```python
from build123d import *

# Parameters (mm, degrees)
SKETCH1_R           = 21
SKETCH1_R_2         = 15.5
SKETCH1_R_3         = 1.5
BOSS_EXTRUDE1_DEPTH = 3
SKETCH2_R           = 2.5
BOSS_EXTRUDE2_DEPTH = 29
CUT_EXTRUDE1_START  = -5
SKETCH3_R           = 1.5
CUT_EXTRUDE1_DEPTH  = 5


with BuildPart() as part:
    # Sketch1 → Boss-Extrude1 (new body)
    with BuildSketch(Plane(origin=(0, 0, 0), x_dir=(1, 0, 0), z_dir=(0, 1, 0))):
        with Locations(Location((0, 0, 0), (0, 0, 270))):
            Circle(SKETCH1_R)
        with Locations(Location((0, 0, 0), (0, 0, 270))):
            Circle(SKETCH1_R_2, mode=Mode.SUBTRACT)
        with Locations(Location((0, 18.25, 0), (0, 0, 270))):
            Circle(SKETCH1_R_3, mode=Mode.SUBTRACT)
        with Locations(Location((12.904698757, 12.904698757, 0), (0, 0, 270))):
            Circle(SKETCH1_R_3, mode=Mode.SUBTRACT)
        with Locations(Location((18.25, 0, 0), (0, 0, 270))):
            Circle(SKETCH1_R_3, mode=Mode.SUBTRACT)
        with Locations(Location((12.904698757, -12.904698757, 0), (0, 0, 270))):
            Circle(SKETCH1_R_3, mode=Mode.SUBTRACT)
        with Locations(Location((0, -18.25, 0), (0, 0, 270))):
            Circle(SKETCH1_R_3, mode=Mode.SUBTRACT)
        with Locations(Location((-12.904698757, -12.904698757, 0), (0, 0, 270))):
            Circle(SKETCH1_R_3, mode=Mode.SUBTRACT)
        with Locations(Location((-18.25, 0, 0), (0, 0, 270))):
            Circle(SKETCH1_R_3, mode=Mode.SUBTRACT)
        with Locations(Location((-12.904698757, 12.904698757, 0), (0, 0, 270))):
            Circle(SKETCH1_R_3, mode=Mode.SUBTRACT)
    extrude(amount=BOSS_EXTRUDE1_DEPTH)

    # Sketch2 → Boss-Extrude2 (add)
    with BuildSketch(Plane(origin=(0, 3, 0), x_dir=(1, 0, 0), z_dir=(0, 1, 0))):
        with Locations(Location((0, 18.25, 0), (0, 0, 90))):
            Circle(SKETCH2_R)
        with Locations(Location((18.25, 0, 0), (0, 0, 90))):
            Circle(SKETCH2_R)
        with Locations(Location((0, -18.25, 0), (0, 0, 90))):
            Circle(SKETCH2_R)
        with Locations(Location((-18.25, 0, 0), (0, 0, 90))):
            Circle(SKETCH2_R)
    extrude(amount=BOSS_EXTRUDE2_DEPTH)

    # Sketch3 → Cut-Extrude1 (cut)
    with BuildSketch(Plane(origin=(0, 32, 0), x_dir=(1, 0, 0), z_dir=(0, 1, 0)).offset(CUT_EXTRUDE1_START)):
        with Locations(Location((18.25, 0, 0), (0, 0, 270))):
            Circle(SKETCH3_R)
        with Locations(Location((0, 18.25, 0), (0, 0, 270))):
            Circle(SKETCH3_R)
        with Locations(Location((0, -18.25, 0), (0, 0, 270))):
            Circle(SKETCH3_R)
        with Locations(Location((-18.25, 0, 0), (0, 0, 270))):
            Circle(SKETCH3_R)
    extrude(amount=CUT_EXTRUDE1_DEPTH, mode=Mode.SUBTRACT)


solid = part.part
```
The model under review builds one solid part; all positions refer to its coordinate system, in mm. A direction names the side the tool comes from. Give positions to 0.01 mm unless a question says otherwise; leave off trailing zeros. Order: outer loops, then holes, each group sorted by start corner. A loop starts at its lowest first (then second) coordinate and runs counter-clockwise, first axis right, second up. Notation, with made-up numbers: (-3.75, -18) - (24.25, -18) arc R12 ccw to (24.25, -2) - close; hole circle Ø8 at (14.25, 41). An arc over 180 degrees is marked (long way). Use CSV: the item, a comma, the result in double quotes. Start each with the question number.
Q1. We need section B-B, the plane z = -6.5. Write out the cut boundary in (x, y).
Q2. Tool access review of faces 1 (the cylindrical face through (-14.37, 1.48, 12.58)), 2 (the flat face through (18, 3, 0)), 3 (the flat face through (0, 27, 18)): name each direction out of +Z, -Z, +X, -X, +Y, -Y from which nothing blocks a thin tool from reaching the whole face with its end or side.
Q3. To check wall thickness, follow line 1 along X through (y, z) = (28.4, 0); line 2 along X through (y, z) = (0.9, 0); line 3 along Z through (x, y) = (2, 4.5). State the ranges of each line that lie inside material, in increasing order. Write a range as [from, to].
Q4. Clearance check with flat-ended pins moving along their axes: pin 1 Ø10 at (x, y) = (12.5, 19.5) entering from -Z; pin 2 Ø8 at (y, z) = (26, -2.5) entering from +X; pin 3 Ø1.5 at (x, z) = (18, 0.5) entering from +Y. State where each tip first meets the part, or that it passes through.
Q5. We need section D-D, the plane x = 18.25. Write out the cut boundary in (y, z), and give its area (3 significant figures).
Q6. We need section C-C, the plane y = 13. Write out the cut boundary in (x, z).
Q7. The part is to be moulded in two halves that separate along X. For faces 4 (the flat face through (-15.5, 0, -3.2)), 5 (the cylindrical face through (13.92, 1.48, -14.01)), 6 (the cylindrical face through (-0.11, 17.297, 20.748)), say which applies: +X half, -X half, draft (parallel to the pull), parting line (faces both ways), or undercut.
Outcome:
1,outline,"(-19.97, 0) - (-14.07, 0) - (-14.07, 3) - (-19.97, 3) - close; (14.07, 0) - (19.97, 0) - (19.97, 3) - (14.07, 3) - close"
2,face 1,"+Y, -Y"
2,face 2,"-Y"
2,face 3,"+Y"
3,line 1,"x = [-20.75, -19.75], [-16.75, -15.75], [15.75, 16.75], [19.75, 20.75]"
3,line 2,"x = [-21, -19.75], [-16.75, -15.5], [15.5, 16.75], [19.75, 21]"
3,line 3,"z = [-19.75, -16.75], [16.75, 19.75]"
4,pin 1,"stops at z = -2.38"
4,pin 2,"stops at x = 20.75"
4,pin 3,"stops at y = 27"
5,outline,"(0, -10.39) - (3, -10.39) - (3, -2.5) - (32, -2.5) - (32, -1.5) - (27, -1.5) - (27, 1.5) - (32, 1.5) - (32, 2.5) - (3, 2.5) - (3, 10.39) - (0, 10.39) - (0, 1.5) - (3, 1.5) - (3, -1.5) - (0, -1.5) - close"
5,area,"183 mm^2"
6,outline,"circle Ø5 at (-18.25, 0); circle Ø5 at (0, -18.25); circle Ø5 at (0, 18.25); circle Ø5 at (18.25, 0)"
7,face 4,"draft"
7,face 5,"undercut"
7,face 6,"parting line"
